from build123d import *

# Parameters (mm, degrees)
BOSS_EXTRUDE1_DEPTH = 38.1
SKETCH2_W           = 260.312588867
SKETCH2_H           = 25.4
CUT_EXTRUDE1_DEPTH  = 206.003825783
SKETCH3_R           = 1.905
CUT_EXTRUDE2_DEPTH  = 206.003825783


with BuildPart() as part:
    # Sketch1 → Boss-Extrude1 (new body)
    with BuildSketch(Plane.XY):
        with BuildLine():
            Line((0, 0), (0, 19.05))
            Line((0, 19.05), (141.01618732, 19.05))
            add(Edge.make_bspline(
                [(191.161472393, 38.021436866), (157.754291932, 137.325067756), (141.01618732, 19.05)],
                knots=[5.354344466, 5.354344466, 5.354344466, 7.54928898, 7.54928898, 7.54928898], degree=2, weights=[1, 0.455847413, 1]))
            Line((191.161472393, 38.021436866), (180.098192457, 33.90003112))
            add(Edge.make_bspline(
                [(180.098192457, 33.90003112), (152.4, 132.820472934), (152.4, 0)],
                knots=[5.442998148, 5.442998148, 5.442998148, 7.853981634, 7.853981634, 7.853981634], degree=2, weights=[1, 0.357233797, 1]))
            Line((152.4, 0), (0, 0))
        make_face()
    extrude(amount=BOSS_EXTRUDE1_DEPTH)

    # Sketch2 → Cut-Extrude1 (cut, through all)
    with BuildSketch(Plane.XZ):
        with Locations((155.556294433, 19.05)):
            Rectangle(SKETCH2_W, SKETCH2_H)
    extrude(amount=-CUT_EXTRUDE1_DEPTH, mode=Mode.SUBTRACT)

    # Sketch3 → Cut-Extrude2 (cut, through all)
    with BuildSketch(Plane.XY.offset(38.1)):
        with Locations((69.85, 9.525)):
            Circle(SKETCH3_R)
    extrude(amount=-CUT_EXTRUDE2_DEPTH, mode=Mode.SUBTRACT)


solid = part.part
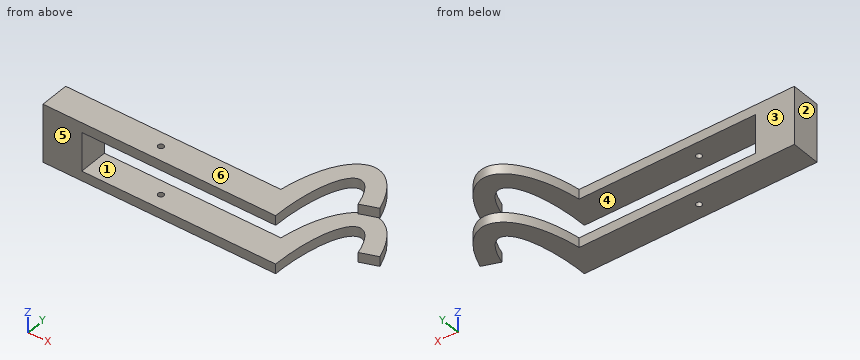
Part model, mm, in its own coordinate system. Face numbers are marked on the shaded views. A direction names the side the tool comes from. Give positions to 0.01 mm unless a question says otherwise; leave off trailing zeros. Order: outer loops, then holes, each group sorted by start corner. A loop starts at its lowest first (then second) coordinate and runs counter-clockwise, first axis right, second up. Notation, with made-up numbers: (-12, 5) -> (-4, 5) arc R27 cw to (-4, 33) -> close; hole circle Ø3 at (61.25, 7.5). An arc over 180 degrees is marked (long way). Use one line per item in the form item = value.
(1) Saw through at C-C (z = 21.5). Write the cut outline in (x, y).
Solution:
outline = (0, 0) -> (25.4, 0) -> (25.4, 19.05) -> (0, 19.05) -> close
(2) Flat gauge pins, fed straight in: P1, Ø2, axis at y = 18.5, z = 27.5, coming from the -X side; P2, Ø8, axis at x = 129, z = 4, coming from the +Y side; P3, Ø9.5, axis at y = 9, z = 25, coming from the +X side. Where does each tip first touch, or does it go through?
Solution:
P1 = 0
P2 = 19.05
P3 = 25.4
(3) Drill centre lines: line 1 (Y direction, x = 69.85, z = 37.25); line 2 (Z direction, x = 52, y = 5); line 3 (X direction, y = 6, z = 26). Where is each one in solid material? Low to high. Write a range as from..to.
Solution:
line_1 = 0..7.62, 11.43..19.05
line_2 = 0..6.35, 31.75..38.1
line_3 = 0..25.4
(4) Tool access for the marked faces 1, 2 and 3: list every direction of +Z, -Z, +X, -X, +Y, -Y with a clear straight run to the whole face (end or side of a thin tool).
Solution:
face_1 = +X, +Y, -Y
face_2 = +Z, -Z, -X, +Y, -Y
face_3 = +Z, -Z, -X, +Y
(5) Saw through at A-A (x = 91.5). Write the cut outline in (y, z).
Solution:
outline = (0, 0) -> (19.05, 0) -> (19.05, 6.35) -> (0, 6.35) -> close; (0, 31.75) -> (19.05, 31.75) -> (19.05, 38.1) -> (0, 38.1) -> close
(6) Pull direction Z, two halves, no side cores. Call the marked faces 4, 5 and 6: +Z half, -Z half, draft (parallel to the pull), parting line (faces both ways), or undercut.
Solution:
face_4 = undercut
face_5 = draft
face_6 = +Z half
(7) Saw through at B-B (x = 69.85). Write the cut outline in (y, z).
Solution:
outline = (0, 0) -> (7.62, 0) -> (7.62, 6.35) -> (0, 6.35) -> close; (0, 31.75) -> (7.62, 31.75) -> (7.62, 38.1) -> (0, 38.1) -> close; (11.43, 0) -> (19.05, 0) -> (19.05, 6.35) -> (11.43, 6.35) -> close; (11.43, 31.75) -> (19.05, 31.75) -> (19.05, 38.1) -> (11.43, 38.1) -> close
